```python
from build123d import *

# Parameters (mm, degrees)
SKETCH6_R           = 12.7
SKETCH6_R_2         = 0.9115
BOSS_EXTRUDE3_DEPTH = 1.5875


with BuildPart() as part:
    # Sketch6 → Boss-Extrude3 (new body)
    # profile 1 of 2: a face of its own
    with BuildSketch(Plane.XY):
        Circle(SKETCH6_R)
        with BuildLine():
            ThreePointArc((6.269554118, 8.885849209), (0, 10.875), (-6.269554118, 8.885849209))
            Line((-6.269554118, 8.885849209), (-5.055813485, 7.672108576))
            ThreePointArc((-5.055813485, 7.672108576), (-5.055813485, 5.055813485), (-7.672108576, 5.055813485))
            Line((-7.672108576, 5.055813485), (-8.885849209, 6.269554118))
            ThreePointArc((-8.885849209, 6.269554118), (-10.875, 0), (-8.885849209, -6.269554118))
            Line((-8.885849209, -6.269554118), (-7.672108576, -5.055813485))
            ThreePointArc((-7.672108576, -5.055813485), (-5.055813485, -5.055813485), (-5.055813485, -7.672108576))
            Line((-5.055813485, -7.672108576), (-6.269554118, -8.885849209))
            ThreePointArc((-6.269554118, -8.885849209), (0, -10.875), (6.269554118, -8.885849209))
            Line((6.269554118, -8.885849209), (5.055813485, -7.672108576))
            ThreePointArc((5.055813485, -7.672108576), (5.055813485, -5.055813485), (7.672108576, -5.055813485))
            Line((7.672108576, -5.055813485), (8.885849209, -6.269554118))
            ThreePointArc((8.885849209, -6.269554118), (10.875, 0), (8.885849209, 6.269554118))
            Line((8.885849209, 6.269554118), (7.672108576, 5.055813485))
            ThreePointArc((7.672108576, 5.055813485), (5.055813485, 5.055813485), (5.055813485, 7.672108576))
            Line((5.055813485, 7.672108576), (6.269554118, 8.885849209))
        make_face(mode=Mode.SUBTRACT)
    # profile 2 of 2: a face of its own
    with BuildSketch(Plane.XY):
        with BuildLine():
            Line((5.055813485, 7.672108576), (6.269554118, 8.885849209))
            ThreePointArc((6.269554118, 8.885849209), (0, 10.875), (-6.269554118, 8.885849209))
            Line((-6.269554118, 8.885849209), (-5.055813485, 7.672108576))
            ThreePointArc((-5.055813485, 7.672108576), (-5.055813485, 5.055813485), (-7.672108576, 5.055813485))
            Line((-7.672108576, 5.055813485), (-8.885849209, 6.269554118))
            ThreePointArc((-8.885849209, 6.269554118), (-10.875, 0), (-8.885849209, -6.269554118))
            Line((-8.885849209, -6.269554118), (-7.672108576, -5.055813485))
            ThreePointArc((-7.672108576, -5.055813485), (-5.055813485, -5.055813485), (-5.055813485, -7.672108576))
            Line((-5.055813485, -7.672108576), (-6.269554118, -8.885849209))
            ThreePointArc((-6.269554118, -8.885849209), (0, -10.875), (6.269554118, -8.885849209))
            Line((6.269554118, -8.885849209), (5.055813485, -7.672108576))
            ThreePointArc((5.055813485, -7.672108576), (5.055813485, -5.055813485), (7.672108576, -5.055813485))
            Line((7.672108576, -5.055813485), (8.885849209, -6.269554118))
            ThreePointArc((8.885849209, -6.269554118), (10.875, 0), (8.885849209, 6.269554118))
            Line((8.885849209, 6.269554118), (7.672108576, 5.055813485))
            ThreePointArc((7.672108576, 5.055813485), (5.055813485, 5.055813485), (5.055813485, 7.672108576))
        make_face()
        with Locations((0, 9.000000134)):
            Circle(SKETCH6_R_2, mode=Mode.SUBTRACT)
        with Locations((9.000000134, 0)):
            Circle(SKETCH6_R_2, mode=Mode.SUBTRACT)
        with Locations((0, -9.000000134)):
            Circle(SKETCH6_R_2, mode=Mode.SUBTRACT)
        with Locations((-9.000000134, 0)):
            Circle(SKETCH6_R_2, mode=Mode.SUBTRACT)
        with BuildLine():
            ThreePointArc((-1.663855614, -6.850845531), (4.985102807, -4.985102807), (6.850845531, 1.663855614))
            ThreePointArc((6.850845531, 1.663855614), (6.830865544, 1.714608205), (6.79791666, 1.758075393))
            Line((6.79791666, 1.758075393), (1.758075393, 6.79791666))
            ThreePointArc((1.758075393, 6.79791666), (1.714608205, 6.830865544), (1.663855614, 6.850845531))
            ThreePointArc((1.663855614, 6.850845531), (-4.985102807, 4.985102807), (-6.850845531, -1.663855614))
            ThreePointArc((-6.850845531, -1.663855614), (-6.830865544, -1.714608205), (-6.79791666, -1.758075393))
            Line((-6.79791666, -1.758075393), (-1.758075393, -6.79791666))
            ThreePointArc((-1.758075393, -6.79791666), (-1.714608205, -6.830865544), (-1.663855614, -6.850845531))
        make_face(mode=Mode.SUBTRACT)
    extrude(amount=BOSS_EXTRUDE3_DEPTH)


solid = part.part
```
The model under review builds one solid part; all positions refer to its coordinate system, in mm. A direction names the side the tool comes from. Round coordinates to 2 decimals unless told otherwise and drop trailing zeros. Loops run counter-clockwise (first coordinate to the right, second up) from the corner with the lowest first, then second, coordinate; pieces in that order, holes last.
Item 1: Mouldability with a two-part tool opening along X and no side actions: class faces 3 (the face through (-4.91, 5.06, 0.78)), 4 (the face through (-2.75, -12.4, 0.78)), 5 (the face through (5.5, -5.5, 1.588)) as released by +X, released by -X, zero draft, split by the parting line, or undercut.
Determined:
face 3: undercut
face 4: split by the parting line
face 5: zero draft
Item 2: Take a section at C-C (z = 1). Write out the cut boundary in (x, y), then the cut area to 3 significant figures.
Determined:
outline: circle Ø25.4 at (0, 0); hole circle Ø1.82 at (-9, 0); hole (-6.85, -1.66) arc R0.2 ccw to (-6.8, -1.76) - (-1.76, -6.8) arc R0.2 ccw to (-1.66, -6.85) arc R7.05 ccw to (6.85, 1.66) arc R0.2 ccw to (6.8, 1.76) - (1.76, 6.8) arc R0.2 ccw to (1.66, 6.85) arc R7.05 ccw to start; hole circle Ø1.82 at (0, -9); hole circle Ø1.82 at (0, 9); hole circle Ø1.82 at (9, 0)
area: 350 mm2
Item 3: For line 1 (Y direction, x = 0, z = 0.6); line 2 (Y direction, x = -9, z = 0.9); line 3 (X direction, y = -1.25, z = 1.35), list the stretches that pass through material, from the lowest coordinate up.
Determined:
line 1: y = -12.7 to -9.91, -8.09 to -7.05, 7.05 to 8.09, 9.91 to 12.7
line 2: y = -8.96 to -0.91, 0.91 to 8.96
line 3: x = -12.64 to -6.94, 6.94 to 12.64
Item 4: Take a section at D-D (x = 9). Write out the cut boundary in (y, z).
Determined:
outline: (-8.96, 0) - (-0.91, 0) - (-0.91, 1.59) - (-8.96, 1.59) - close; (0.91, 0) - (8.96, 0) - (8.96, 1.59) - (0.91, 1.59) - close
Item 5: For faces 1 (the face through (4.313, 4.243, 0.783)), 2 (the face through (5.5, -5.5, 0)), list the 3-axis set-ups (+Z, -Z, +X, -X, +Y, -Y) from which the entire face can be reached by the end or side of a thin tool; tool diameter is ignored.
Determined:
face 1: +Z, -Z
face 2: -Z, +X, -X, +Y, -Y
Item 6: Take a section at A-A (x = 0). Write out the cut boundary in (y, z), then the cut area to 3 significant figures.
Determined:
outline: (-12.7, 0) - (-9.91, 0) - (-9.91, 1.59) - (-12.7, 1.59) - close; (-8.09, 0) - (-7.05, 0) - (-7.05, 1.59) - (-8.09, 1.59) - close; (7.05, 0) - (8.09, 0) - (8.09, 1.59) - (7.05, 1.59) - close; (9.91, 0) - (12.7, 0) - (12.7, 1.59) - (9.91, 1.59) - close
area: 12.2 mm2
